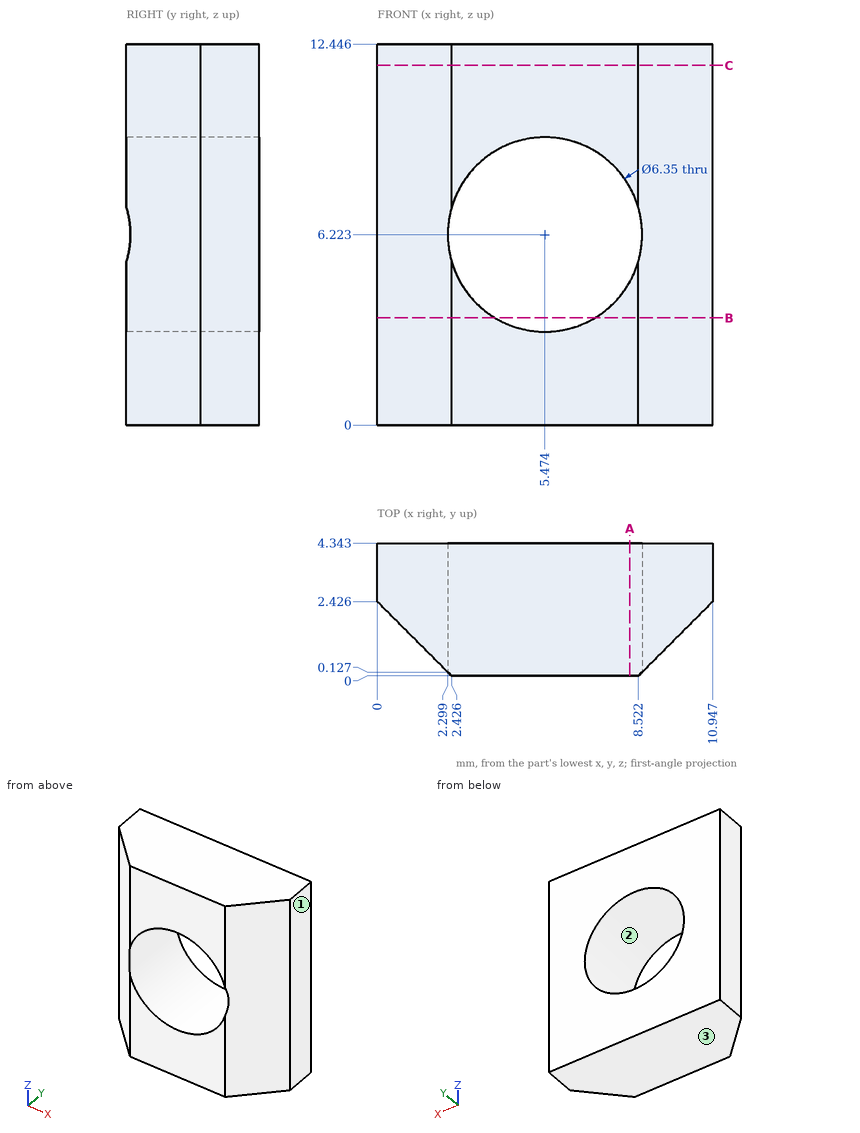
Geometry check sheet. Reference: drawing and pictorial views, mm from the part's lowest x, y, z. Coordinates: 2 decimals unless noted, no trailing zeros. Order: outer loops, then holes, each group sorted by start corner. A loop starts at its lowest first (then second) coordinate and runs counter-clockwise, first axis right, second up. Notation, with made-up numbers: (-25, 81) - (-10, 81) arc R17 ccw to (-10, 113) - close; hole circle Ø10 at (45.25, 39.25). An arc over 180 degrees is marked (long way). Answer in a Markdown table with one row per item. Add a question column.
1) Cross-section at A-A, the plane x = 8.25. Record the cut outline in (y, z).
2) Release check for a two-part mould opening along Z. For the marked faces 1, 2 and 3 record: +Z half, -Z half, draft (parallel to the pull), parting line (faces both ways), or undercut.
3) Cross-section at B-B, the plane z = 3.5. Record the cut outline in (x, y) (1 decimal).
4) Cross-section at C-C, the plane z = 11.75. Record the cut outline in (x, y) (1 decimal).
5) Material ranges on line 1 along X through (y, z) = (0.3, 8) (1 decimal); line 2 along X through (y, z) = (0.8, 8.5) (1 decimal); line 3 along Z through (x, y) = (8, 0.75) (1 decimal), recorded low to high. Write a range as [from, to].
6) Gauge pin test, flat end, axial feed: P1, Ø2, axis at y = 3.5, z = 5.5, coming from the -X side. Record the tip position at first contact, or that the pin passes through.
Check result:
| question | item | result |
|---|---|---|
| 1 | outline | (0, 0) - (4.34, 0) - (4.34, 4.68) - (0, 4.68) - close; (0, 7.76) - (4.34, 7.76) - (4.34, 12.45) - (0, 12.45) - close |
| 2 | face 1 | draft |
| 2 | face 2 | undercut |
| 2 | face 3 | -Z half |
| 3 | outline | (0, 2.4) - (2.4, 0) - (3.8, 0) - (3.8, 4.3) - (0, 4.3) - close; (7.1, 0) - (8.5, 0) - (10.9, 2.4) - (10.9, 4.3) - (7.1, 4.3) - close |
| 4 | outline | (0, 2.4) - (2.4, 0) - (8.5, 0) - (10.9, 2.4) - (10.9, 4.3) - (0, 4.3) - close |
| 5 | line 1 | x = [2.1, 2.8], [8.1, 8.8] |
| 5 | line 2 | x = [1.6, 3.3], [7.7, 9.3] |
| 5 | line 3 | z = [0, 4.3], [8.1, 12.4] |
| 6 | P1 | stops at x = 0 |
